from build123d import *

# Parameters (mm, degrees)
SKETCH_W        = 65
SKETCH_H        = 20
SKETCH_R        = 4.125
PAD_DEPTH       = 3.25
SKETCH001_W     = 20
SKETCH001_H     = 3.25
PAD001_DEPTH    = 20
SKETCH002_R     = 1.5
SKETCH002_W     = 2
SKETCH002_H     = 2
POCKET_DEPTH    = 5
FILLET_R        = 5
SKETCH003_R     = 3
POCKET001_DEPTH = 1
SKETCH004_R     = 4.75
POCKET002_DEPTH = 1


with BuildPart() as part:
    # Sketch → Pad (new body)
    with BuildSketch(Plane.XY):
        with Locations((32.5, 10)):
            Rectangle(SKETCH_W, SKETCH_H)
        with Locations((15, 10)):
            Circle(SKETCH_R, mode=Mode.SUBTRACT)
        with Locations((50, 10)):
            Circle(SKETCH_R, mode=Mode.SUBTRACT)
        with Locations((35, 10)):
            Circle(SKETCH_R, mode=Mode.SUBTRACT)
    extrude(amount=PAD_DEPTH)

    # Sketch001 (on DatumPlane) → Pad001 (join)
    with BuildSketch(Plane(origin=(0, 0, 0), x_dir=(0, -1, 0), z_dir=(-1, 0, 0))):
        with Locations((-10, 1.625)):
            Rectangle(SKETCH001_W, SKETCH001_H)
    extrude(amount=PAD001_DEPTH)

    # Sketch002 (on DatumPlane) → Pocket (cut)
    with BuildSketch(Plane.XY.offset(3.25)):
        with Locations((-14.5625, 10)):
            Circle(SKETCH002_R)
        with Locations((59.5625, 10)):
            Circle(SKETCH002_R)
        with Locations((-4.375, 10)):
            Rectangle(SKETCH002_W, SKETCH002_H)
    extrude(amount=-POCKET_DEPTH, mode=Mode.SUBTRACT)

    # Fillet
    fillet_edges = [part.edges().sort_by_distance(p)[0] for p in [
        (-20, 20, 1.625),
        (-20, 0, 1.625),
        (65, 0, 1.625),
        (65, 20, 1.625),
    ]]
    fillet(fillet_edges, radius=FILLET_R)

    # Sketch003 (on DatumPlane) → Pocket001 (cut)
    with BuildSketch(Plane.XY.offset(3.25)):
        with Locations((-14.5625, 10)):
            Circle(SKETCH003_R)
        with Locations((59.5625, 10)):
            Circle(SKETCH003_R)
    extrude(amount=-POCKET001_DEPTH, mode=Mode.SUBTRACT)

    # Sketch004 (on DatumPlane) → Pocket002 (cut)
    with BuildSketch(Plane(origin=(0, 0, 0), x_dir=(1, 0, 0), z_dir=(0, 0, -1))):
        with Locations((-4.375, -10)):
            Circle(SKETCH004_R)
    extrude(amount=-POCKET002_DEPTH, mode=Mode.SUBTRACT)


solid = part.part
The listing builds one solid part. Answer for the finished solid, in the listing's coordinates (mm). A direction names the side the tool comes from. Coordinates: 2 decimals unless noted, no trailing zeros. Write each loop counter-clockwise with the first axis right and the second up, starting at its lowest first coordinate (ties: lowest second). Pieces come first, ordered by that corner, then holes. Notation, with made-up numbers: (-5, 6.25) - (1, 6.25) arc R26 ccw to (1, 41.25) - close; hole circle Ø11 at (85, 73). An arc over 180 degrees is marked (long way). Put each result on its own line as item: value.
1. Find the intervals of material crossed by line 1 along Y through (x, z) = (50, 0.8) (3 decimals); line 2 along X through (y, z) = (8.25, 1.7); line 3 along X through (y, z) = (13, 0.7), in increasing order. Write a range as from..to.
Answer sheet:
line 1: y = 0..5.875, 14.125..20
line 2: x = -20..11.26, 18.74..31.26, 38.74..46.26, 53.74..65
line 3: x = -20..-8.06, -0.69..12.17, 17.83..32.17, 37.83..47.17, 52.83..65
2. The part is cut by section B-B on y = 10. State how many separate pieces and enclosed holes the cut face has, plus the area to 3 significant figures.
Answer sheet:
separate pieces: 7
enclosed holes: 0
area: 156 mm^2
3. The part is cut by section A-A on x = 35. Give the vertices of the cut face in (y, z) (3 decimals).
Answer sheet:
outline: (0, 0) - (5.875, 0) - (5.875, 3.25) - (0, 3.25) - close; (14.125, 0) - (20, 0) - (20, 3.25) - (14.125, 3.25) - close
4. The part is cut by section C-C on x = 50.5. Give the vertices of the cut face in (y, z), plus the area to 3 significant figures.
Answer sheet:
outline: (0, 0) - (5.91, 0) - (5.91, 3.25) - (0, 3.25) - close; (14.09, 0) - (20, 0) - (20, 3.25) - (14.09, 3.25) - close
area: 38.4 mm^2
5. Determine the mould class of faces 1 (the face through (23, 20, 2)), 2 (the face through (65, 10, 2)), 3 (the face through (60.993, 10.451, 1.141)) for opening direction Y: pulls with the +Y half, pulls with the -Y half, needs draft (parallel to the pull), parting line crosses it, or undercut.
Answer sheet:
face 1: pulls with the +Y half
face 2: needs draft
face 3: undercut
6. The part is cut by section D-D on x = -6.5. Give the vertices of the cut face in (y, z).
Answer sheet:
outline: (0, 0) - (5.75, 0) - (5.75, 1) - (14.25, 1) - (14.25, 0) - (20, 0) - (20, 3.25) - (0, 3.25) - close
7. A tool of negligible diameter and unlimited length cuts with its end or side. For faces 4 (the face through (-17.56, 10.13, 2.76)), 5 (the face through (0.156, 8.573, 0.493)), 6 (the face through (-4, 11, 2)), from which of +Z, -Z, +X, -X, +Y, -Y can it reach the whole face along a straight path? Write none if from no direction.
Answer sheet:
face 4: +Z
face 5: -Z
face 6: +Z, -Z
8. Flat-ended cylindrical pins translate along their axes: pin 1 Ø2 at (x, y) = (6.5, 11.5) entering from -Z; pin 2 Ø3 at (x, y) = (-15.5, 10) entering from +Z; pin 3 Ø3 at (x, y) = (-2, 8.5) entering from -Z. Find the tip coordinate at first contact, or state that the pin passes through.
Answer sheet:
pin 1: stops at z = 0
pin 2: stops at z = 2.25
pin 3: stops at z = 1
